```python
from build123d import *

# Parameters (mm, degrees)
ENL_V_MAT_EXTRU_1_REACH      = 28.401
ESQUISSE3_W                  = 2
ESQUISSE3_H                  = 15.856728551
ESQUISSE4_R                  = 2.95
ENL_V_MAT_EXTRU_2_DEPTH      = 6
ENL_V_MAT_EXTRU_2_DRAFT      = -3
R_P_TITION_CIRCULAIRE4_COUNT = 12
ESQUISSE5_W                  = 5.287177124
ESQUISSE5_H                  = 1.2
ENL_V_MAT_EXTRU_3_DEPTH      = 2.5


with BuildPart() as part:
    # Esquisse1 → Révolution1 (revolve)
    with BuildSketch(Plane.XY):
        Polygon((0, 0), (-7.5, 0), (-6.5, 18), (0, 18), align=None)
    revolve(axis=Axis((0, 18, 0), (0, -1, 0)))

    # Enlèv. mat.-Extru.1: from a cone face, 28.401 long prism both ways, kept between that surface and its translate by the depth
    enl_v_mat_extru_1_start = Plane(origin=(0, 9.428364, 0), z_dir=(0, -1, 0)) * Cone(4.983024111, 8.969379889, 71.754404, mode=Mode.PRIVATE)
    enl_v_mat_extru_1_end = Plane(origin=(0, 9.428364, -0.2), z_dir=(0, -1, 0)) * Cone(4.983024111, 8.969379889, 71.754404, mode=Mode.PRIVATE)
    # Esquisse3 → Enlèv. mat.-Extru.1 (cut, from a surface)
    with BuildSketch(Plane.XY.offset(10), mode=Mode.PRIVATE) as enl_v_mat_extru_1_sk1:
        with Locations((0, 9.428364275)):
            Rectangle(ESQUISSE3_W, ESQUISSE3_H)
    enl_v_mat_extru_1_tool1 = extrude(enl_v_mat_extru_1_sk1.sketch, amount=ENL_V_MAT_EXTRU_1_REACH, both=True, mode=Mode.PRIVATE)
    enl_v_mat_extru_1 = ((enl_v_mat_extru_1_tool1 & enl_v_mat_extru_1_start) - enl_v_mat_extru_1_end).solids().sort_by_distance((0, 9.428364, 6.803862))[0]
    add(enl_v_mat_extru_1, mode=Mode.SUBTRACT)


with BuildPart() as enl_v_mat_extru_2_tool:
    # Esquisse4 → Enlèv. mat.-Extru.2 (with draft: the straight prism first)
    with BuildSketch(Plane.XZ):
        Circle(ESQUISSE4_R)
    extrude(amount=-ENL_V_MAT_EXTRU_2_DEPTH)
    # Enlèv. mat.-Extru.2: the draft: its side faces are tilted about the plane it starts from
    enl_v_mat_extru_2_sides = [enl_v_mat_extru_2_tool.faces().sort_by_distance(p)[0] for p in [
        (-2.95, 3, 0),
    ]]
    draft(enl_v_mat_extru_2_sides, Plane.XZ, ENL_V_MAT_EXTRU_2_DRAFT)


with BuildPart() as part_1:
    add(part.part)

    # Enlèv. mat.-Extru.2: cut by enl_v_mat_extru_2_tool
    add(enl_v_mat_extru_2_tool.part, mode=Mode.SUBTRACT)

    # Répétition circulaire4: Enlèv. mat.-Extru.1 ×12 about axis
    r_p_tition_circulaire4_axis = Axis((0, 0, 0), (0, 1, 0))
    for i in range(1, R_P_TITION_CIRCULAIRE4_COUNT):
        add(enl_v_mat_extru_1.rotate(r_p_tition_circulaire4_axis, i * 360 / R_P_TITION_CIRCULAIRE4_COUNT), mode=Mode.SUBTRACT)

    # Esquisse5 → Enlèv. mat.-Extru.3 (cut)
    with BuildSketch(Plane(origin=(0, 20, 0), x_dir=(1, 0, 0), z_dir=(0, 1, 0))):
        with Locations((-3.828659888, 0)):
            Rectangle(ESQUISSE5_W, ESQUISSE5_H)
    extrude(amount=-ENL_V_MAT_EXTRU_3_DEPTH, mode=Mode.SUBTRACT)


solid = part_1.part
```
Source: CAD feature listing. Evaluate the final solid. Frame: model axes, mm. A direction names the side the tool comes from. Coordinates: 2 decimals unless noted, no trailing zeros. Write each loop counter-clockwise with the first axis right and the second up, starting at its lowest first coordinate (ties: lowest second). Pieces come first, ordered by that corner, then holes. Notation, with made-up numbers: M -8,81.5 L 30,81.5 A26 ccw 30,95.5 Z; hole C -37,72.25 d6. An arc over 180 degrees is marked long. Answer as a JSON object with one key per item and string values.
1. Ray query, L1, parallel to Z at x = -2, y = 2.5; L2, parallel to Z at x = -2.5, y = 2.5; L3, parallel to Y at x = -0.75, z = 0.75. Return the intervals inside material, ascending.
Evaluation:
{"L1": "-7.08 to -1.99, 1.99 to 7.08", "L2": "-6.92 to -1.3, 1.3 to 6.92", "L3": "6 to 18"}
2. Contact query for flat-ended pins moving along their axis: P1, Ø1, axis at x = 3, y = 6.5, coming from the +Z side; P2, Ø4, axis at y = 2.5, z = 1, coming from the +X side; P3, Ø0.9, axis at x = -7, y = 6, coming from the +Z side. Output: stop coordinate, or through.
Evaluation:
{"P1": "z = 6.69", "P2": "x = 7.46", "P3": "z = 2.69"}
3. Access query for faces 1 (the conical face through (-6.782, 9.317, 0.015)), 2 (the conical face through (6.782, 9.317, -0.015)). Directions: +Z, -Z, +X, -X, +Y, -Y. A direction counts if a zero-diameter tool reaches every point of the face in a straight line with its end or side. Return the directions, or none.
Evaluation:
{"face 1": "-X", "face 2": "+X"}
4. Cut plane A-A on x = 0. Output: boundary loops of the cut face in (y, z), plus the area to 3 significant figures.
Evaluation:
{"outline": "M 0,-7.5 L 1.5,-7.42 L 1.5,-7.22 L 17.36,-6.34 L 17.36,-6.54 L 18,-6.5 L 18,6.5 L 17.36,6.54 L 17.36,6.34 L 1.5,7.22 L 1.5,7.42 L 0,7.5 L 0,2.95 L 6,2.64 L 6,-2.64 L 0,-2.95 Z", "area": "212 mm^2"}
